Answer from the drawing. Dimensions are ordinates in mm from the lowest x, y and z of the part. A direction names the side the tool comes from. Coordinates: 2 decimals unless noted, no trailing zeros. Order: outer loops, then holes, each group sorted by start corner. A loop starts at its lowest first (then second) coordinate and runs counter-clockwise, first axis right, second up. Notation, with made-up numbers: (-12, 11) - (6, 11) arc R27 cw to (6, 34) - close; hole circle Ø11 at (83.5, -2). An arc over 180 degrees is marked (long way). One line per item, written item: value. Start each with the question number.
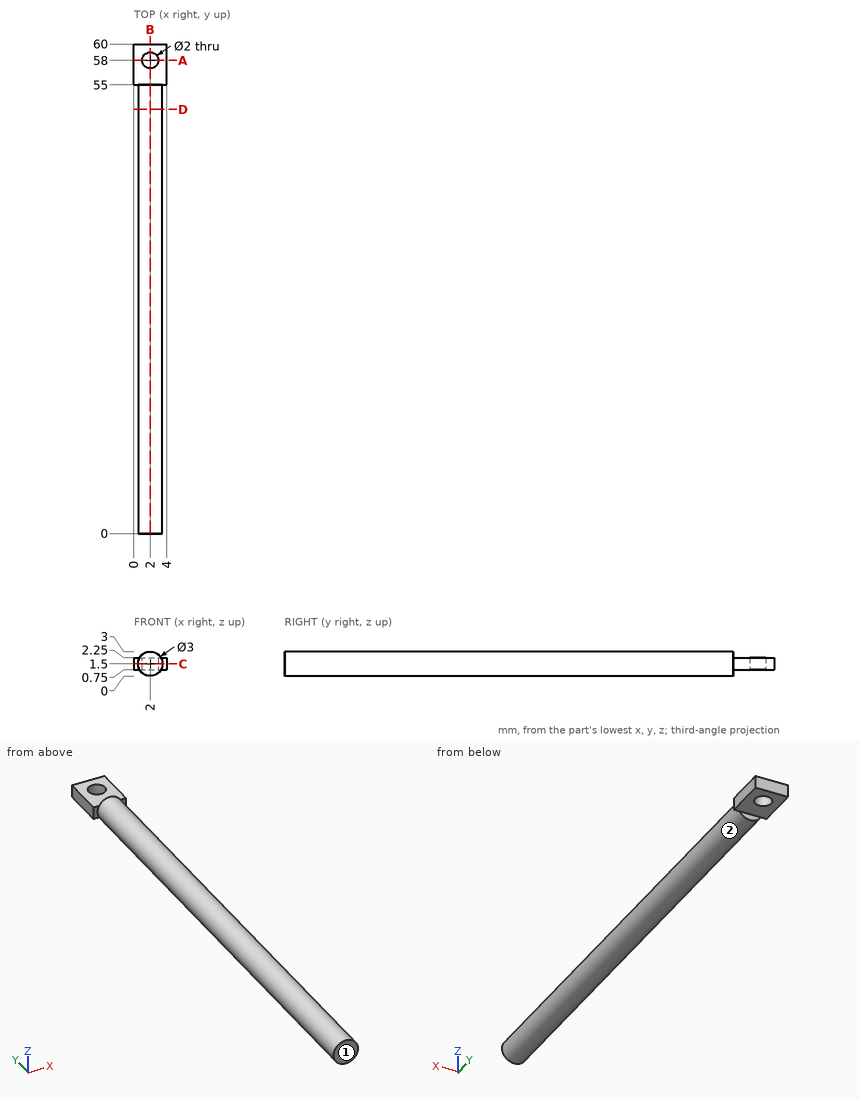
(1) Flat-ended cylindrical pins translate along their axes: pin 1 Ø1.5 at (y, z) = (43, 2) entering from -X; pin 2 Ø0.6 at (x, z) = (3.5, 1.5) entering from -Y; pin 3 Ø1.2 at (x, y) = (2, 58) entering from +Z (3 decimals). Find the tip coordinate at first contact, or state that the pin passes through.
(2) Consider probe 1 along Y at (x, z) = (2, 1.2); probe 2 along Y at (x, z) = (2.8, 2.3); probe 3 along X at (y, z) = (47, 1.45). Determine where each line is inside the solid, lowest interval first.
(3) The part is cut by section C-C on z = 1.5. Determine the outline of the cut face in (x, y), plus the area to 3 significant figures.
(4) For the marked faces 1 and 2, determine the directions among +Z, -Z, +X, -X, +Y, -Y from which every point of the face is accessible in a straight line to the end or side of a thin tool.
(5) The part is cut by section A-A on y = 58. Determine the outline of the cut face in (x, z).
(6) The part is cut by section B-B on x = 2. Determine the outline of the cut face in (y, z), plus the area to 4 significant figures.
(7) The part is cut by section D-D on y = 52. Determine the outline of the cut face in (x, z), plus the area to 3 significant figures.
Completed:
1. pin 1: stops at x = 0.5
1. pin 2: stops at y = 0
1. pin 3: passes through
2. probe 1: y = 0 to 57, 59 to 60
2. probe 2: y = 0 to 55
2. probe 3: x = 0.5 to 3.5
3. outline: (0, 55) - (0.5, 55) - (0.5, 0) - (3.5, 0) - (3.5, 55) - (4, 55) - (4, 60) - (0, 60) - close; hole circle Ø2 at (2, 58)
3. area: 182 mm2
4. face 1: +Z, -Z, +X, -X, -Y
4. face 2: -Y
5. outline: (0, 0.75) - (1, 0.75) - (1, 2.25) - (0, 2.25) - close; (3, 0.75) - (4, 0.75) - (4, 2.25) - (3, 2.25) - close
6. outline: (0, 0) - (55, 0) - (55, 0.75) - (57, 0.75) - (57, 2.25) - (55, 2.25) - (55, 3) - (0, 3) - close; (59, 0.75) - (60, 0.75) - (60, 2.25) - (59, 2.25) - close
6. area: 169.5 mm2
7. outline: circle Ø3 at (2, 1.5)
7. area: 7.07 mm2
